Can you work these out from the model? Positions are in its coordinate system, mm. Face numbers are marked on the shaded views. Round coordinates to 2 decimals unless told otherwise and drop trailing zeros. Loops run counter-clockwise (first coordinate to the right, second up) from the corner with the lowest first, then second, coordinate; pieces in that order, holes last. Notation, with made-up numbers: M 66,14 L 70,14 A15 cw 70,43 Z; hole C 82.25,86.5 d9. An arc over 180 degrees is marked long. Answer as CSV lines item,"result".
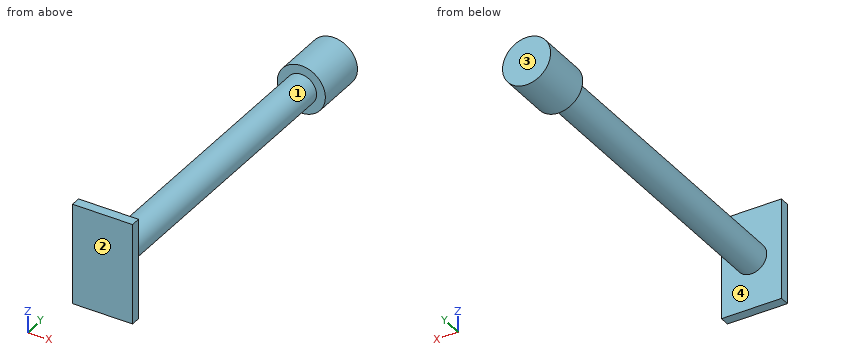
from build123d import *

# Parameters (mm, degrees)
SKETCH1_R           = 7.493
BOSS_EXTRUDE1_DEPTH = 152.4
SKETCH2_W           = 29.464
SKETCH2_H           = 49.53
BOSS_EXTRUDE2_DEPTH = 4.7625
SKETCH3_R           = 11.811
BOSS_EXTRUDE3_DEPTH = 25.4


with BuildPart() as part:
    # Sketch1 → Boss-Extrude1 (new body)
    with BuildSketch(Plane(origin=(0, 0, 0), x_dir=(1, 0, 0), z_dir=(0, 1, 0))):
        with Locations(Location((0, 0, 0), (0, 0, 90))):
            Circle(SKETCH1_R)
    extrude(amount=BOSS_EXTRUDE1_DEPTH)

    # Sketch2 → Boss-Extrude2 (add)
    with BuildSketch(Plane.XZ):
        Rectangle(SKETCH2_W, SKETCH2_H)
    extrude(amount=BOSS_EXTRUDE2_DEPTH)

    # Sketch3 → Boss-Extrude3 (add)
    with BuildSketch(Plane(origin=(0, 152.4, 0), x_dir=(1, 0, 0), z_dir=(0, 1, 0))):
        with Locations(Location((0, 0, 0), (0, 0, 270))):
            Circle(SKETCH3_R)
    extrude(amount=BOSS_EXTRUDE3_DEPTH)


solid = part.part
Item 1: Will these pins go through, and if not, where does the flat tip stop? pin 1 (4 mm diameter, centred on y = 21.5, z = -4, fed in from +X); pin 2 (12 mm diameter, centred on x = -11.5, y = 87.5, fed in from -Z); pin 3 (5 mm diameter, centred on x = -11, z = 7, fed in from +Y); pin 4 (4 mm diameter, centred on x = 9.5, z = -14.5, fed in from +Y).
Output:
pin 1,"stops at x = 7.22"
pin 2,"stops at z = -5.09"
pin 3,"stops at y = 177.8"
pin 4,"stops at y = 0"
Item 2: If we section it at B-B on x = 0: Write out the boundary of the cut face in (y, z) (1 decimal), then the cut area to 3 significant figures.
Output:
outline,"M -4.8,-24.8 L 0,-24.8 L 0,-7.5 L 152.4,-7.5 L 152.4,-11.8 L 177.8,-11.8 L 177.8,11.8 L 152.4,11.8 L 152.4,7.5 L 0,7.5 L 0,24.8 L -4.8,24.8 Z"
area,"3,120 mm2"
Item 3: We'd pull the mould along Y, two halves only. Please class the marked faces 1, 2, 3 and 4: released by +Y, released by -Y, zero draft, split by the parting line, or undercut.
Output:
face 1,"undercut"
face 2,"released by -Y"
face 3,"released by +Y"
face 4,"undercut"
Item 4: If we section it at C-C on y = 115.5: Write out the boundary of the cut face in (x, z).
Output:
outline,"C 0,0 d14.99"
Item 5: If we section it at A-A on z = 0: Write out the boundary of the cut face in (x, y), then the cut area to 3 significant figures.
Output:
outline,"M -14.73,-4.76 L 14.73,-4.76 L 14.73,0 L 7.49,0 L 7.49,152.4 L 11.81,152.4 L 11.81,177.8 L -11.81,177.8 L -11.81,152.4 L -7.49,152.4 L -7.49,0 L -14.73,0 Z"
area,"3,020 mm2"
Item 6: If we section it at D-D on z = 17: Write out the boundary of the cut face in (x, y).
Output:
outline,"M -14.73,-4.76 L 14.73,-4.76 L 14.73,0 L -14.73,0 Z"
Item 7: If I drill on line 1 along Y through (x, z) = (-11.5, -2.5); line 2 along Y through (x, z) = (-2.75, 19.5); line 3 along Z through (x, y) = (0.5, 65.5), over which ranges is the centre line in solid material (lowest first)? Write a range as from..to.
Output:
line 1,"y = -4.76..0, 152.4..177.8"
line 2,"y = -4.76..0"
line 3,"z = -7.48..7.48"
